Answer from the drawing. Dimensions are ordinates in mm from the lowest x, y and z of the part. A direction names the side the tool comes from. Coordinates: 2 decimals unless noted, no trailing zeros. Write each loop counter-clockwise with the first axis right and the second up, starting at its lowest first coordinate (ties: lowest second). Pieces come first, ordered by that corner, then holes.
(1) The part is cut by section B-B, the plane y = 18. Determine the outline of the cut face in (x, z), and give its area (4 significant figures).
(2) Determine the mould class of the marked faces 1, 2 and 3 for opening direction X: pulls with the +X half, pulls with the -X half, needs draft (parallel to the pull), parting line crosses it, or undercut.
(3) The part is cut by section C-C, the plane x = 4. Determine the outline of the cut face in (y, z).
(4) Straight lines are drawn through the part: line 1 along X through (y, z) = (9.5, 27.5); line 2 along Z through (x, y) = (7.75, 57.5). For each, find the intervals that lie inside material, in ascending order.
(5) The part is cut by section A-A, the plane z = 9.5. Determine the outline of the cut face in (x, y), and give its area (3 significant figures).
(6) Given pin 1 (5 mm diameter, centred on x = 8, y = 40.5, fed in from -Z), flat-ended and moving along its own axis, determine where the tip first touches the part or whether it passes through.
(7) Which of the six approach directions +Z, -Z, +X, -X, +Y, -Y give full straight-line access (tool end or side, diameter ignored) to the marked faces 4 and 5?
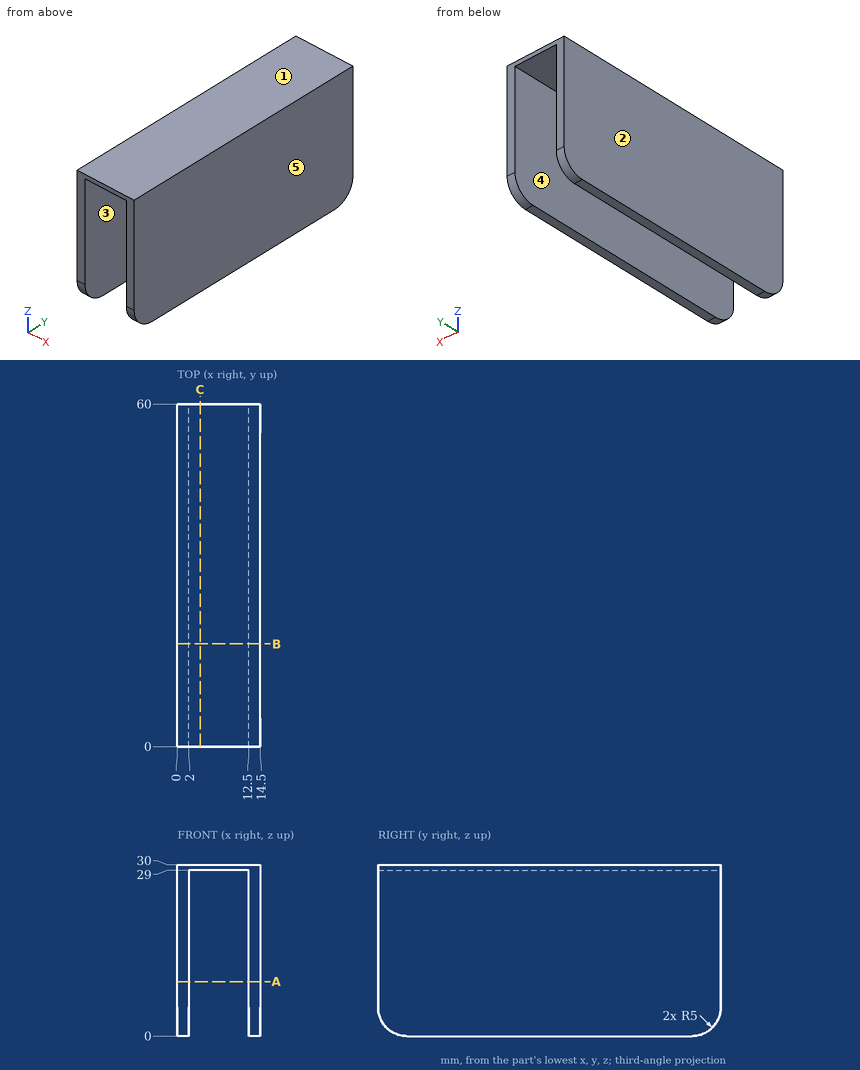
Computed:
1. outline: (0, 0) - (2, 0) - (2, 29) - (12.5, 29) - (12.5, 0) - (14.5, 0) - (14.5, 30) - (0, 30) - close
1. area: 130.5 mm2
2. face 1: needs draft
2. face 2: pulls with the -X half
2. face 3: undercut
3. outline: (0, 29) - (60, 29) - (60, 30) - (0, 30) - close
4. line 1: x = 0 to 2, 12.5 to 14.5
4. line 2: z = 29 to 30
5. outline: (0, 0) - (2, 0) - (2, 60) - (0, 60) - close; (12.5, 0) - (14.5, 0) - (14.5, 60) - (12.5, 60) - close
5. area: 240 mm2
6. pin 1: stops at z = 29
7. face 4: -Z, +Y, -Y
7. face 5: +Z, -Z, +X, +Y, -Y
